from build123d import *

# Parameters (mm, degrees)
BOSS_EXTRUDE1_DEPTH = 2.25
CUT_EXTRUDE1_DEPTH  = 32.519835025
FILLET1_R           = 0.75
BOSS_EXTRUDE2_DEPTH = 2.25
BOSS_EXTRUDE4_DEPTH = 4.5
FILLET2_R           = 1
CUT_EXTRUDE4_DEPTH  = 5
BOSS_EXTRUDE5_START = -2.25
BOSS_EXTRUDE5_DEPTH = 4.5
SKETCH12_W          = 11.535913892
SKETCH12_H          = 0.5
CUT_EXTRUDE5_DEPTH  = 32.519835168


with BuildPart() as part:
    # Sketch1 → Boss-Extrude1 (new, symmetric)
    with BuildSketch(Plane(origin=(0, 0, 0), x_dir=(0, 0, -1), z_dir=(1, 0, 0))):
        Polygon((17.5, 4.025), (17.5, 4.95), (17.5, 8.301357795), (17.5, 8.5), (29, 8.5), (29, -11.5), (17.5, -11.5), (17.5, -8.673247977), (17.5, -5.2), (17.5, -4.025), (23.25, -4.025), (23.25, 4.025), align=None)
    extrude(amount=BOSS_EXTRUDE1_DEPTH, both=True)

    # Sketch4 → Cut-Extrude1 (cut, through all)
    with BuildSketch(Plane.ZY.offset(2.25)):
        with BuildLine():
            Line((-26.625, -11.5), (-26.625, -9.452368755))
            ThreePointArc((-26.625, -9.452368755), (-26.25, -6.5), (-25.875, -9.452368755))
            Line((-25.875, -9.452368755), (-25.875, -11.5))
            Line((-25.875, -11.5), (-26.625, -11.5))
        make_face()
        with BuildLine():
            Line((-20.625, -9.452368755), (-20.625, -11.5))
            Line((-20.625, -11.5), (-19.875, -11.5))
            Line((-19.875, -11.5), (-19.875, -9.452368755))
            ThreePointArc((-19.875, -9.452368755), (-20.25, -6.5), (-20.625, -9.452368755))
        make_face()
    extrude(amount=-CUT_EXTRUDE1_DEPTH, mode=Mode.SUBTRACT)

    # Fillet1
    fillet1_edges = [part.edges().sort_by_distance(p)[0] for p in [
        (0, -4.025, -23.25),
        (0, 4.025, -23.25),
    ]]
    fillet(fillet1_edges, radius=FILLET1_R)

    # Sketch2 → Boss-Extrude2 (add, symmetric)
    with BuildSketch(Plane(origin=(0, 0, 0), x_dir=(0, 0, -1), z_dir=(1, 0, 0))):
        with BuildLine():
            Line((1.7, -6.45), (16.25, -6.45))
            ThreePointArc((16.25, -6.45), (17.133883476, -6.083883476), (17.5, -5.2))
            Line((17.5, -5.2), (17.5, -8.673247977))
            ThreePointArc((17.5, -8.673247977), (17.136039688, -7.776350438), (16.25, -7.38670191))
            add(Edge.make_bspline(
                [(16.25, -7.38670191), (15.982544989, -7.378993429), (15.453928293, -7.363553213), (14.397933299, -7.332164796), (13.361703255, -7.29957206), (12.100876768, -7.258861503), (10.975898138, -7.220164867), (9.768608213, -7.176905715), (8.611498431, -7.132461764), (7.424019565, -7.084024767), (6.255327605, -7.032148986), (5.075409432, -6.975000615), (3.903033551, -6.911058587), (2.727587922, -6.837381628), (1.722719604, -6.759660724), (0.954287884, -6.683217964), (0.456400256, -6.610639739), (0.237084283, -6.56505431), (0.137087499, -6.537027737), (0.087321771, -6.519206998), (0.060111975, -6.507310883), (0.043000809, -6.498417374), (0.030678751, -6.490921905), (0.01600081, -6.480451435), (0.005229873, -6.469720378), (0.000815287, -6.459042222), (0, -6.45)],
                knots=[0.090617463, 0.090617463, 0.090617463, 0.090617463, 0.090617463, 0.156221583, 0.221825702, 0.287429821, 0.35303394, 0.41863806, 0.484242179, 0.549846298, 0.615450417, 0.681054537, 0.746658656, 0.812262775, 0.877866892, 0.943220604, 0.971682344, 0.984222879, 0.990100446, 0.993094331, 0.994839978, 0.995992112, 0.996718592, 0.997392575, 0.998059613, 1, 1, 1, 1, 1], degree=4))
            Line((0, -6.45), (-1.7, -6.45))
            Line((-1.7, -6.45), (-1.7, -4.45))
            ThreePointArc((-1.7, -4.45), (0, -2.75), (1.7, -4.45))
            Line((1.7, -4.45), (1.7, -6.45))
        make_face()
        with BuildLine():
            Line((17.5, 4.95), (17.5, 8.301357795))
            ThreePointArc((17.5, 8.301357795), (17.135773003, 7.406119792), (16.25, 7.019443472))
            add(Edge.make_bspline(
                [(16.25, 7.019443472), (15.987531738, 7.01282569), (15.470119802, 6.999607493), (14.430987801, 6.972604073), (13.4161389, 6.944724509), (12.177418763, 6.909818433), (11.074067802, 6.876745116), (9.888671574, 6.839769393), (8.753245319, 6.801895235), (7.587539532, 6.760659557), (6.440473735, 6.716696676), (5.282208442, 6.668364938), (4.131254265, 6.614778963), (2.976099529, 6.553298089), (1.935166314, 6.486657721), (1.112090632, 6.419330464), (0.550531612, 6.355136747), (0.26288649, 6.306396396), (0.144856484, 6.278329018), (0.090076692, 6.261554801), (0.061106748, 6.250555216), (0.043474041, 6.242594857), (0.030984848, 6.235965644), (0.016604026, 6.227042793), (0.005627844, 6.21781856), (0.000998515, 6.208209958), (0, 6.2)],
                knots=[0.090678734, 0.090678734, 0.090678734, 0.090678734, 0.090678734, 0.15510723, 0.219535726, 0.283964222, 0.348392717, 0.412821213, 0.477249709, 0.541678205, 0.606106701, 0.670535197, 0.734963692, 0.799392188, 0.863820683, 0.928249179, 0.967999033, 0.983460374, 0.990010293, 0.993269409, 0.995072657, 0.996228288, 0.996922821, 0.997582549, 0.998234329, 1, 1, 1, 1, 1], degree=4))
            Line((0, 6.2), (-1.7, 6.2))
            Line((-1.7, 6.2), (-1.7, 4.2))
            ThreePointArc((-1.7, 4.2), (0, 2.5), (1.7, 4.2))
            Line((1.7, 4.2), (1.7, 6.2))
            Line((1.7, 6.2), (16.25, 6.2))
            ThreePointArc((16.25, 6.2), (17.133883476, 5.833883476), (17.5, 4.95))
        make_face()
    extrude(amount=BOSS_EXTRUDE2_DEPTH, both=True)

    # Sketch3 → Boss-Extrude4 (add, through all)
    with BuildSketch(Plane.ZY.offset(2.25)):
        with BuildLine():
            Line((1.7, -6.45), (-1.690848844, -6.752163217))
            add(Edge.make_bspline(
                [(0, -6.45), (-0.000815287, -6.459042222), (-0.005229873, -6.469720378), (-0.01600081, -6.480451435), (-0.030678751, -6.490921905), (-0.043000809, -6.498417374), (-0.060111975, -6.507310883), (-0.087321771, -6.519206998), (-0.137087499, -6.537027737), (-0.237084283, -6.56505431), (-0.456400256, -6.610639739), (-0.842629924, -6.666941327), (-1.204799072, -6.706915262), (-1.511345405, -6.736167418), (-1.690848844, -6.752163217)],
                knots=[0.090617463, 0.090617463, 0.090617463, 0.090617463, 0.090617463, 0.09255785, 0.093224888, 0.093898872, 0.094625351, 0.095777486, 0.097523132, 0.100517018, 0.106394584, 0.118935119, 0.14739686, 0.187580696, 0.187580696, 0.187580696, 0.187580696, 0.187580696], degree=4))
            Line((0, -6.45), (1.7, -6.45))
        make_face()
        with BuildLine():
            Line((0, 6.2), (1.7, 6.2))
            Line((1.7, 6.2), (-1.70169721, 6.465184862))
            add(Edge.make_bspline(
                [(-1.70169721, 6.465184862), (-1.588493346, 6.45635987), (-1.29771245, 6.43266583), (-0.938114175, 6.399442625), (-0.550531612, 6.355136747), (-0.26288649, 6.306396396), (-0.144856484, 6.278329018), (-0.090076692, 6.261554801), (-0.061106748, 6.250555216), (-0.043474041, 6.242594857), (-0.030984848, 6.235965644), (-0.016604026, 6.227042793), (-0.005627844, 6.21781856), (-0.000998515, 6.208209958), (0, 6.2)],
                knots=[0.902915454, 0.902915454, 0.902915454, 0.902915454, 0.902915454, 0.928249179, 0.967999033, 0.983460374, 0.990010293, 0.993269409, 0.995072657, 0.996228288, 0.996922821, 0.997582549, 0.998234329, 1, 1, 1, 1, 1], degree=4))
        make_face()
    extrude(amount=-BOSS_EXTRUDE4_DEPTH)

    # Fillet2
    fillet2_edges = [part.edges().sort_by_distance(p)[0] for p in [
        (0, -6.45, -1.7),
        (0, -6.45, 1.7),
        (0, 6.2, 1.7),
        (0, 6.2, -1.7),
    ]]
    fillet(fillet2_edges, radius=FILLET2_R)

    # Sketch6 → Cut-Extrude4 (cut, symmetric)
    with BuildSketch(Plane(origin=(0, 0, 0), x_dir=(0, 0, -1), z_dir=(1, 0, 0))):
        with BuildLine():
            Line((-1.6125, -4.3375), (-1.696273489, -4.3375))
            Line((-1.696273489, -4.3375), (-1.696273489, -2.65))
            Line((-1.696273489, -2.65), (1.696273489, -2.65))
            Line((1.696273489, -2.65), (1.696273489, -4.3375))
            Line((1.696273489, -4.3375), (1.6125, -4.3375))
            ThreePointArc((1.6125, -4.3375), (0, -5.95), (-1.6125, -4.3375))
        make_face()
        with BuildLine():
            Line((1.612242467, 4.083682007), (1.696015956, 4.083682007))
            Line((1.696015956, 4.083682007), (1.696015956, 2.396182007))
            Line((1.696015956, 2.396182007), (-1.696015956, 2.396182007))
            Line((-1.696015956, 2.396182007), (-1.696015956, 4.083682007))
            Line((-1.696015956, 4.083682007), (-1.612242467, 4.083682007))
            ThreePointArc((-1.612242467, 4.083682007), (0, 5.725), (1.612242467, 4.083682007))
        make_face()
    extrude(amount=CUT_EXTRUDE4_DEPTH, both=True, mode=Mode.SUBTRACT)

    # Sketch9 → Boss-Extrude5 (add)
    with BuildSketch(Plane(origin=(0, 0, 0), x_dir=(0, 0, -1), z_dir=(1, 0, 0)).offset(BOSS_EXTRUDE5_START)):
        with BuildLine():
            Line((-1.696273489, -4.3375), (-1.8825, -4.3375))
            Line((-1.8825, -4.3375), (-1.8825, -5.065291012))
            ThreePointArc((-1.8825, -5.065291012), (-1.767426598, -5.679381925), (-1.437821002, -6.210145232))
            ThreePointArc((-1.437821002, -6.210145232), (-1.63215369, -5.89721165), (-1.7, -5.535148811))
            Line((-1.7, -5.535148811), (-1.7, -4.45))
            ThreePointArc((-1.7, -4.45), (-1.699068117, -4.393719149), (-1.696273489, -4.3375))
        make_face()
        with BuildLine():
            Line((1.8825, -4.3375), (1.8825, -5.890593975))
            ThreePointArc((1.8825, -5.890593975), (1.911190263, -6.034829666), (1.992893219, -6.157106781))
            ThreePointArc((1.992893219, -6.157106781), (1.776120467, -5.832683432), (1.7, -5.45))
            Line((1.7, -5.45), (1.7, -4.45))
            ThreePointArc((1.7, -4.45), (1.699068117, -4.393719149), (1.696273489, -4.3375))
            Line((1.696273489, -4.3375), (1.6125, -4.3375))
            ThreePointArc((1.6125, -4.3375), (1.565557971, -3.951255919), (1.427464973, -3.5875))
            Line((1.427464973, -3.5875), (1.8825, -3.5875))
            Line((1.8825, -3.5875), (1.8825, -4.3375))
        make_face()
        with BuildLine():
            Line((1.696015956, 4.083682007), (1.882242467, 4.083682007))
            Line((1.882242467, 4.083682007), (1.882242467, 5.639972236))
            ThreePointArc((1.882242467, 5.639972236), (1.910999661, 5.78454441), (1.992893219, 5.907106781))
            ThreePointArc((1.992893219, 5.907106781), (1.776120467, 5.582683432), (1.7, 5.2))
            Line((1.7, 5.2), (1.7, 4.2))
            ThreePointArc((1.7, 4.2), (1.699003697, 4.141806899), (1.696015956, 4.083682007))
        make_face()
        with BuildLine():
            Line((-1.882242467, 4.083682007), (-1.882242467, 4.809550575))
            ThreePointArc((-1.882242467, 4.809550575), (-1.766204889, 5.424085171), (-1.434071123, 5.95399521))
            ThreePointArc((-1.434071123, 5.95399521), (-1.631147443, 5.639565509), (-1.7, 5.274922618))
            Line((-1.7, 5.274922618), (-1.7, 4.2))
            ThreePointArc((-1.7, 4.2), (-1.699003697, 4.141806899), (-1.696015956, 4.083682007))
            Line((-1.696015956, 4.083682007), (-1.612242467, 4.083682007))
            ThreePointArc((-1.612242467, 4.083682007), (-1.587589378, 3.830159396), (-1.523321299, 3.583682007))
            Line((-1.523321299, 3.583682007), (-1.882242467, 3.583682007))
            Line((-1.882242467, 3.583682007), (-1.882242467, 4.083682007))
        make_face()
    extrude(amount=BOSS_EXTRUDE5_DEPTH)

    # Sketch12 → Cut-Extrude5 (cut, through all)
    with BuildSketch(Plane.ZY.offset(2.25)):
        with Locations((-23.232043054, 8.25)):
            Rectangle(SKETCH12_W, SKETCH12_H)
    extrude(amount=-CUT_EXTRUDE5_DEPTH, mode=Mode.SUBTRACT)


solid = part.part
The listing builds one solid part. Answer for the finished solid, in the listing's coordinates (mm). A direction names the side the tool comes from. Give positions to 0.01 mm unless a question says otherwise; leave off trailing zeros. Loops run counter-clockwise (first coordinate to the right, second up) from the corner with the lowest first, then second, coordinate; pieces in that order, holes last.
Item 1: Determine the mould class of faces 1 (the flat face through (-0.031, 6.367, -0.445)), 2 (the flat face through (0, 0, -23.25)), 3 (the flat face through (0, -10, -19.875)) for opening direction Y: +Y half, -Y half, draft (parallel to the pull), parting line (faces both ways), or undercut.
Derived:
face 1: +Y half
face 2: undercut
face 3: draft
Item 2: A cutting plane is placed at C-C (z = -21). Give the vertices of the cut face in (x, y) (3 decimals).
Derived:
outline: (-2.25, -11.5) - (2.25, -11.5) - (2.25, -9.299) - (-2.25, -9.299) - close; (-2.25, -6.701) - (2.25, -6.701) - (2.25, -4.025) - (-2.25, -4.025) - close; (-2.25, 4.025) - (2.25, 4.025) - (2.25, 8) - (-2.25, 8) - close
Item 3: A cutting plane is placed at D-D (y = -0.5). Give the vertices of the cut face in (x, z), then the cut area to 3 significant figures.
Derived:
outline: (-2.25, -29) - (2.25, -29) - (2.25, -23.25) - (-2.25, -23.25) - close
area: 25.9 mm2
Item 4: A cutting plane is placed at A-A (z = -1). Give the vertices of the cut face in (x, y).
Derived:
outline: (-2.25, -6.69) - (2.25, -6.69) - (2.25, -5.6) - (-2.25, -5.6) - close; (-2.25, 5.38) - (2.25, 5.38) - (2.25, 6.41) - (-2.25, 6.41) - close
Item 5: A cutting plane is placed at B-B (y = -8.25). Give the vertices of the cut face in (x, z), then the cut area to 3 significant figures.
Derived:
outline: (-2.25, -29) - (2.25, -29) - (2.25, -27.73) - (-2.25, -27.73) - close; (-2.25, -24.77) - (2.25, -24.77) - (2.25, -21.73) - (-2.25, -21.73) - close; (-2.25, -18.77) - (2.25, -18.77) - (2.25, -17.43) - (-2.25, -17.43) - close
area: 25.4 mm2
Item 6: Find the intervals of material crossed by line 1 along Z through (x, y) = (1.85, 4.25); line 2 along Y through (x, z) = (0.6, -16); line 3 along Z through (x, y) = (1.35, -10.25) (3 decimals), in increasing order.
Derived:
line 1: z = -29 to -17.5, -1.88 to -1.61, 1.61 to 1.88
line 2: y = -7.38 to -6.45, 6.2 to 7.01
line 3: z = -29 to -26.625, -25.875 to -20.625, -19.875 to -17.5
Item 7: Each of these flat-tipped pins is pushed along its axis until it touches: pin 1 Ø2.5 at (x, y) = (0, -10.5) entering from +Z; pin 2 Ø2 at (x, y) = (-0.5, -0.5) entering from +Z; pin 3 Ø2 at (x, z) = (1, -11) entering from -Y (3 decimals). Where does it stop, or does it pass through?
Derived:
pin 1: stops at z = -17.5
pin 2: stops at z = -23.25
pin 3: stops at y = -7.255
Item 8: A tool of negligible diameter and unlimited length cuts with its end or side. For faces 4 (the flat face through (2.25, -2, -24)), 5 (the cylindrical face through (0.031, 5.844, -17.124)), 6 (the flat face through (0, -10, -25.875)), from which of +Z, -Z, +X, -X, +Y, -Y can it reach the whole face along a straight path? Write none if from no direction.
Derived:
face 4: +Z, -Z, +X, +Y, -Y
face 5: +X, -X
face 6: +X, -X, -Y
